The listing builds one solid part. Answer for the finished solid, in the listing's coordinates (mm). A direction names the side the tool comes from. Give positions to 0.01 mm unless a question says otherwise; leave off trailing zeros. Write each loop counter-clockwise with the first axis right and the second up, starting at its lowest first coordinate (ties: lowest second). Pieces come first, ordered by that corner, then holes. Notation, with made-up numbers: (-26, 43.5) -> (10, 43.5) arc R25 ccw to (10, 76.5) -> close; hole circle Ø3 at (34.5, 76). An arc over 180 degrees is marked (long way). Put each result on its own line as item: value. Start each with the question number.
1) A cutting plane is placed at C-C (y = 2). Write down the section's boundary in (x, z).
2) A cutting plane is placed at A-A (x = 70). Write down the section's boundary in (y, z), then the cut area to 3 significant figures.
3) For faces 1 (the flat face through (94, 3, 8.1)), 2 (the cylindrical face through (9.798, 16.537, 0.507)), 3 (the flat face through (96, 15, 3)), determine the directions among +Z, -Z, +X, -X, +Y, -Y from which every point of the face is accessible in a straight line to the end or side of a thin tool.
4) A cutting plane is placed at D-D (y = 15). Write down the section's boundary in (x, z).
5) Find the intervals of material crossed by line 1 along Z through (x, y) = (129, 6); line 2 along X through (y, z) = (16.5, 2.5); line 3 along Y through (x, z) = (164.5, 8.5), in increasing order. Write a range as from..to.
6) Flat-ended cylindrical pins translate along their axes: pin 1 Ø3.5 at (x, y) = (92, 3) entering from -Z; pin 2 Ø4 at (x, y) = (60, 19) entering from +Z; pin 3 Ø4.5 at (x, y) = (180, 15) entering from +Z. Find the tip coordinate at first contact, or state that the pin passes through.
7) A cutting plane is placed at B-B (z = 6.5). Write down the section's boundary in (x, y), then the cut area to 3 significant figures.
8) For a pull along Y with two mould halves and no side action, classify faces 4 (the flat face through (94, 30, 5)), 5 (the flat face through (94, 27, 10)), 6 (the flat face through (96, 7, 9)) as released by +Y, released by -Y, zero draft, split by the parting line, or undercut.
from build123d import *

# Parameters (mm, degrees)
SKETCH1_W           = 190
SKETCH1_H           = 30
BOSS_EXTRUDE1_DEPTH = 10
SKETCH2_W           = 7
SKETCH2_H           = 16
CUT_EXTRUDE1_DEPTH  = 191
CUT_EXTRUDE2_REACH  = 32
SKETCH4_R           = 2.05
SKETCH4_R_2         = 1.55
SKETCH4_R_3         = 4
CUT_EXTRUDE3_DEPTH  = 4
CHAMFER1_SIZE       = 2
CHAMFER2_SIZE       = 2


with BuildPart() as part:
    # Sketch1 → Boss-Extrude1 (new body)
    with BuildSketch(Plane.XY):
        with Locations((95, 15)):
            Rectangle(SKETCH1_W, SKETCH1_H)
    extrude(amount=BOSS_EXTRUDE1_DEPTH)

    # Sketch2 → Cut-Extrude1 (cut, through all)
    with BuildSketch(Plane(origin=(190, 0, 0), x_dir=(0, 0, -1), z_dir=(1, 0, 0))):
        with Locations((-6.5, 15)):
            Rectangle(SKETCH2_W, SKETCH2_H)
    extrude(amount=-CUT_EXTRUDE1_DEPTH, mode=Mode.SUBTRACT)

    # Sketch3 → Cut-Extrude2 (cut, up to next)
    with BuildSketch(Plane.XZ, mode=Mode.PRIVATE) as cut_extrude2_sk1:
        with BuildLine():
            Line((7.5, 8.1), (182.5, 8.1))
            ThreePointArc((182.5, 8.1), (184.1, 6.5), (182.5, 4.9))
            Line((182.5, 4.9), (7.5, 4.9))
            ThreePointArc((7.5, 4.9), (5.9, 6.5), (7.5, 8.1))
        make_face()
    cut_extrude2_tool1 = extrude(cut_extrude2_sk1.sketch, amount=-CUT_EXTRUDE2_REACH, mode=Mode.PRIVATE) & part.part
    add(cut_extrude2_tool1.solids().sort_by_distance((95, 0, 6.5))[0], mode=Mode.SUBTRACT)

    # Sketch4 → Cut-Extrude3 (cut, through all)
    with BuildSketch(Plane.XY.offset(3)):
        with Locations((180, 15)):
            Circle(SKETCH4_R)
        with Locations((10, 15)):
            Circle(SKETCH4_R_2)
        with Locations((70, 15)):
            Circle(SKETCH4_R_3)
    extrude(amount=-CUT_EXTRUDE3_DEPTH, mode=Mode.SUBTRACT)

    # Chamfer1
    chamfer1_edges = [part.edges().sort_by_distance(p)[0] for p in [
        (177.95, 15, 3),
    ]]
    chamfer(chamfer1_edges, length=CHAMFER1_SIZE)

    # Chamfer2
    chamfer2_edges = [part.edges().sort_by_distance(p)[0] for p in [
        (8.45, 15, 3),
    ]]
    chamfer(chamfer2_edges, length=CHAMFER2_SIZE)


solid = part.part
Reply:
1. outline: (0, 0) -> (190, 0) -> (190, 10) -> (0, 10) -> close; hole (7.5, 4.9) -> (182.5, 4.9) arc R1.6 ccw to (182.5, 8.1) -> (7.5, 8.1) arc R1.6 ccw to start
2. outline: (0, 0) -> (11, 0) -> (11, 3) -> (7, 3) -> (7, 4.9) -> (0, 4.9) -> close; (0, 8.1) -> (7, 8.1) -> (7, 10) -> (0, 10) -> close; (19, 0) -> (30, 0) -> (30, 10) -> (23, 10) -> (23, 3) -> (19, 3) -> close
2. area: 142 mm2
3. face 1: -Y
3. face 2: +Z, -Z
3. face 3: +Z, +X, -X
4. outline: (0, 0) -> (8.45, 0) -> (8.45, 1) -> (6.45, 3) -> (0, 3) -> close; (11.55, 0) -> (66, 0) -> (66, 3) -> (13.55, 3) -> (11.55, 1) -> close; (74, 0) -> (177.95, 0) -> (177.95, 1) -> (175.95, 3) -> (74, 3) -> close; (182.05, 0) -> (190, 0) -> (190, 3) -> (184.05, 3) -> (182.05, 1) -> close
5. line 1: z = 0..4.9, 8.1..10
5. line 2: x = 0..7.34, 12.66..66.29, 73.71..176.78, 183.22..190
5. line 3: y = 0..7, 23..30
6. pin 1: stops at z = 0
6. pin 2: stops at z = 3
6. pin 3: stops at z = 1.2
7. outline: (0, 0) -> (5.9, 0) -> (5.9, 7) -> (0, 7) -> close; (0, 23) -> (190, 23) -> (190, 30) -> (0, 30) -> close; (184.1, 0) -> (190, 0) -> (190, 7) -> (184.1, 7) -> close
7. area: 1,410 mm2
8. face 4: released by +Y
8. face 5: zero draft
8. face 6: undercut
